from build123d import *

# Parameters (mm, degrees)
SKETCH1_R                   = 42.545
BOSS_EXTRUDE1_DEPTH         = 15.875
SKETCH2_R                   = 39.3446
SKETCH2_R_2                 = 34.7218
GROOVE_232ORING_DEPTH       = 2.6416
F_1_4_20_TAPPED_HOLE1_D     = 5.1054
F_1_4_20_TAPPED_HOLE1_DEPTH = 7.874
F_1_4_20_TAPPED_HOLE1_TIP   = 1.533816902
SKETCH7_R                   = 4.7625
CUT_EXTRUDE2_DEPTH          = 16.875
SKETCH8_R                   = 1.3589
CUT_EXTRUDE3_DEPTH          = 3.302
CHAMFER1_SIZE               = 0.340295474
CHAMFER1_SIZE2              = 1.27
CHAMFER2_SIZE               = 1.27
FILLET1_R                   = 0.254


with BuildPart() as part:
    # Sketch1 → Boss-Extrude1 (new body)
    with BuildSketch(Plane.XZ):
        Circle(SKETCH1_R)
    extrude(amount=-BOSS_EXTRUDE1_DEPTH)

    # Sketch2 → Groove_232Oring (cut)
    with BuildSketch(Plane.XZ):
        Circle(SKETCH2_R)
        Circle(SKETCH2_R_2, mode=Mode.SUBTRACT)
    extrude(amount=-GROOVE_232ORING_DEPTH, mode=Mode.SUBTRACT)

    # 1/4-20 Tapped Hole1
    with Locations(Plane(origin=(0, 0, 0), x_dir=(-1, 0, 0), z_dir=(0, -1, 0))):
        with Locations((-7.395754214, 27.601330486), (7.395754214, -27.601330486)):
            Hole(F_1_4_20_TAPPED_HOLE1_D / 2, depth=F_1_4_20_TAPPED_HOLE1_DEPTH)
            with Locations((0, 0, -(F_1_4_20_TAPPED_HOLE1_DEPTH + F_1_4_20_TAPPED_HOLE1_TIP / 2))):  # 118° drill point
                Cone(0, F_1_4_20_TAPPED_HOLE1_D / 2, F_1_4_20_TAPPED_HOLE1_TIP, mode=Mode.SUBTRACT)

    # Sketch7 → Cut-Extrude2 (cut, through all)
    with BuildSketch(Plane(origin=(0, 15.875, 0), x_dir=(-1, 0, 0), z_dir=(0, 1, 0))):
        Circle(SKETCH7_R)
    extrude(amount=-CUT_EXTRUDE2_DEPTH, mode=Mode.SUBTRACT)

    # Sketch8 → Cut-Extrude3 (cut)
    with BuildSketch(Plane(origin=(0, 15.875, 0), x_dir=(-1, 0, 0), z_dir=(0, 1, 0))):
        with Locations((-7.1374, 0)):
            Circle(SKETCH8_R)
    extrude(amount=-CUT_EXTRUDE3_DEPTH, mode=Mode.SUBTRACT)

    # Chamfer1
    chamfer1_edges = [part.edges().sort_by_distance(p)[0] for p in [
        (4.7625, 15.875, 0),
    ]]
    chamfer1_side = [part.faces().sort_by_distance(p)[0] for p in [
        (-41.34164568, 15.875, 0),
    ]]
    chamfer(chamfer1_edges, length=CHAMFER1_SIZE, length2=CHAMFER1_SIZE2, reference=chamfer1_side[0])

    # Chamfer2
    chamfer2_edges = [part.edges().sort_by_distance(p)[0] for p in [
        (-42.545, 15.875, 0),
    ]]
    chamfer(chamfer2_edges, length=CHAMFER2_SIZE)

    # Fillet1
    fillet1_edges = [part.edges().sort_by_distance(p)[0] for p in [
        (-39.3446, 2.6416, 0),
        (-34.7218, 2.6416, 0),
        (-39.3446, 0, 0),
        (-34.7218, 0, 0),
    ]]
    fillet(fillet1_edges, radius=FILLET1_R)


solid = part.part
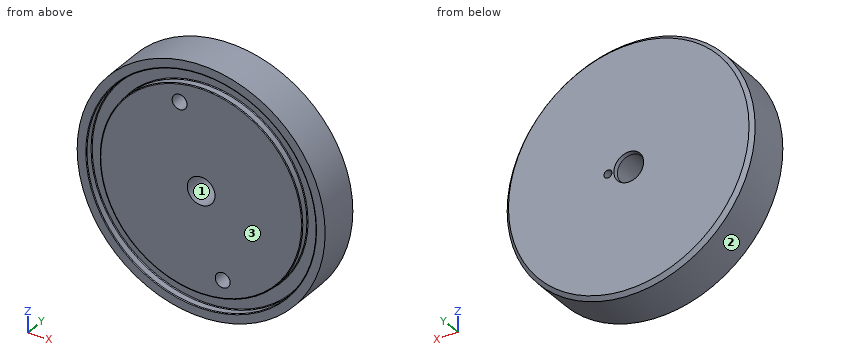
The listing builds one solid part. Answer for the finished solid, in the listing's coordinates (mm). Face numbers are marked on the shaded views. Round coordinates to 2 decimals unless told otherwise and drop trailing zeros. Use a Markdown table: item, result. Add a question column.
1. For a pull along Z with two mould halves and no side action, classify the marked faces 1, 2 and 3 as +Z half, -Z half, draft (parallel to the pull), parting line (faces both ways), or undercut.
2. Consider line 1 (X direction, y = 2, z = -26.5); line 2 (X direction, y = 1.75, z = -5); line 3 (Y direction, x = -35, z = -3.5) (3 decimals). Determine where each line is inside the solid, lowest interval first.
3. Flat-ended cylindrical pins translate along their axes: P1, Ø1.4, axis at x = 7.5, z = 0.5, coming from the +Y side; P2, Ø4.5, axis at x = 7.14, z = 0, coming from the -Y side; P3, Ø4, axis at x = -18.5, y = 5.5, coming from the -Z side; P4, Ø5, axis at x = 33, y = 14, coming from the +Z side. Find the tip coordinate at first contact, or state that the pin passes through.
Reported:
| question | item | result |
|---|---|---|
| 1 | face 1 | undercut |
| 1 | face 2 | parting line |
| 1 | face 3 | draft |
| 2 | line 1 | -33.28 to -29.08, -22.44 to 5.09, 9.7 to 22.44, 29.08 to 33.28 |
| 2 | line 2 | -42.25 to -39.03, -34.36 to 34.36, 39.03 to 42.25 |
| 2 | line 3 | 2.642 to 15.875 |
| 3 | P1 | y = 12.57 |
| 3 | P2 | y = 0 |
| 3 | P3 | z = -39.22 |
| 3 | P4 | z = 29.66 |
